Input: part model. Units: mm. Frame: model coordinates. Round coordinates to 2 decimals unless told otherwise and drop trailing zeros. Loops run counter-clockwise (first coordinate to the right, second up) from the corner with the lowest first, then second, coordinate; pieces in that order, holes last. Notation, with made-up numbers: M 15.25,64 L 65.25,64 A29 ccw 65.25,103 Z; hole C 30,-20.5 d3. An arc over 180 degrees is marked long. Put each result on its own line as item: value. Start each with the question number.
1) Pin query (flat end, axial travel): pin 1 (7.5 mm diameter, centred on x = 0, y = 0, fed in from -Z); pin 2 (3 mm diameter, centred on x = -5.5, z = -35, fed in from +Y); pin 3 (5 mm diameter, centred on y = 1, z = -26.5, fed in from +X); pin 4 (5 mm diameter, centred on y = 3, z = -53.5, fed in from +X). Return the tip coordinate at first contact, or that it passes through.
2) Line query: probe 1 along Y at (x, z) = (0, -47); probe 2 along X at (y, z) = (3, -58); probe 3 along X at (y, z) = (1, -30) (3 decimals). Output: solid intervals per line, ascending.
3) Draft query along X for faces 1 (the face through (4.19, -5.44, -34.44)), 2 (the face through (-3, -6.35, -34)), 3 (the face through (-4.11, -2.41, -34.44)). Return one class per face: +X half, -X half, draft (parallel to the pull), parting line (faces both ways), or undercut.
4) Section A-A on x = 0. Output: boundary loops of the cut face in (y, z).
from build123d import *

# Parameters (mm, degrees)
SKETCH1_R           = 2.9337
BOSS_EXTRUDE1_DEPTH = 69.85


with BuildPart() as part:
    # Sketch1 → Boss-Extrude1 (new body)
    with BuildSketch(Plane(origin=(0, 0, 0), x_dir=(-1, 0, 0), z_dir=(0, 0, -1))):
        with BuildLine():
            Line((-4.70551159, -4.549815043), (-3.666174521, -6.349999904))
            Line((-3.666174521, -6.349999904), (-1.587500385, -6.349999904))
            ThreePointArc((-1.587500385, -6.349999904), (-3.85e-07, -4.762499904), (1.587499615, -6.349999904))
            Line((1.587499615, -6.349999904), (3.666173825, -6.349999904))
            Line((3.666173825, -6.349999904), (4.705510942, -4.54981524))
            ThreePointArc((4.705510942, -4.54981524), (4.124445629, -2.381249907), (6.293010962, -1.800184594))
            Line((6.293010962, -1.800184594), (7.332348079, 7e-08))
            Line((7.332348079, 7e-08), (6.293011217, 1.800184685))
            ThreePointArc((6.293011217, 1.800184685), (4.124445939, 2.381250203), (4.705511457, 4.549815481))
            Line((4.705511457, 4.549815481), (3.666174521, 6.350000222))
            Line((3.666174521, 6.350000222), (1.587500385, 6.350000222))
            ThreePointArc((1.587500385, 6.350000222), (3.85e-07, 4.762500222), (-1.587499615, 6.350000222))
            Line((-1.587499615, 6.350000222), (-3.666173825, 6.350000222))
            Line((-3.666173825, 6.350000222), (-4.705511038, 4.549815614))
            ThreePointArc((-4.705511038, 4.549815614), (-4.124445841, 2.38125025), (-6.293011205, 1.800185053))
            Line((-6.293011205, 1.800185053), (-7.332348419, 4.44e-07))
            Line((-7.332348419, 4.44e-07), (-6.293011423, -1.80018429))
            ThreePointArc((-6.293011423, -1.80018429), (-4.12444613, -2.38124975), (-4.70551159, -4.549815043))
        make_face()
        Circle(SKETCH1_R, mode=Mode.SUBTRACT)
    extrude(amount=BOSS_EXTRUDE1_DEPTH)


solid = part.part
Geometry results:
1. pin 1: stops at z = -69.85
1. pin 2: stops at y = 5.77
1. pin 3: stops at x = 7.33
1. pin 4: stops at x = 7.04
2. probe 1: y = -4.76 to -2.93, 2.93 to 4.76
2. probe 2: x = -3.92 to 3.92
2. probe 3: x = -6.755 to -2.758, 2.758 to 6.755
3. face 1: +X half
3. face 2: draft
3. face 3: undercut
4. outline: M -4.76,-69.85 L -2.93,-69.85 L -2.93,0 L -4.76,0 Z; M 2.93,-69.85 L 4.76,-69.85 L 4.76,0 L 2.93,0 Z
